Part model, mm, in its own coordinate system. Face numbers are marked on the shaded views. A direction names the side the tool comes from. Give positions to 0.01 mm unless a question says otherwise; leave off trailing zeros. Write each loop counter-clockwise with the first axis right and the second up, starting at its lowest first coordinate (ties: lowest second). Pieces come first, ordered by that corner, then holes.
from build123d import *


with BuildPart() as part:
    # Sketch 1 → Revolve 394 (revolve)
    with BuildSketch(Plane.XY, mode=Mode.PRIVATE) as revolve_394_sk:
        Polygon((-12.5, 0), (-12.5, -37.5), (-10, -37.5), (-10, -207.5), (-12.5, -207.5), (-12.5, -227.5), (0, -227.5), (0, -207.591623727), (-8, -207.591623727), (-8, 0), align=None)
    revolve(revolve_394_sk.sketch.rotate(Axis((0, -1459.557248463, 0), (0, 1, 0)), 180), axis=Axis((0, -1459.557248463, 0), (0, 1, 0)))


with BuildPart() as revolve_813_tool:
    # Sketch 3 → Revolve 813 (revolve)
    with BuildSketch(Plane(origin=(0, 0, 0), x_dir=(1, 0, 0), z_dir=(0, 1, 0))):
        Polygon((-60, 10), (-40, 10), (-36, 10), (-36, 12.5), (36, 12.5), (36, 10), (60, 10), (60, 8), (-60, 8), align=None)
    revolve(axis=Axis((60, 0, 0), (1, 0, 0)))


with BuildPart() as part_1:
    add(part.part)


with BuildPart() as part_2:
    # Revolve 813: joined with revolve_813_tool
    add(part_1.part.fuse(revolve_813_tool.part, tol=0.00001))


solid = part_2.part
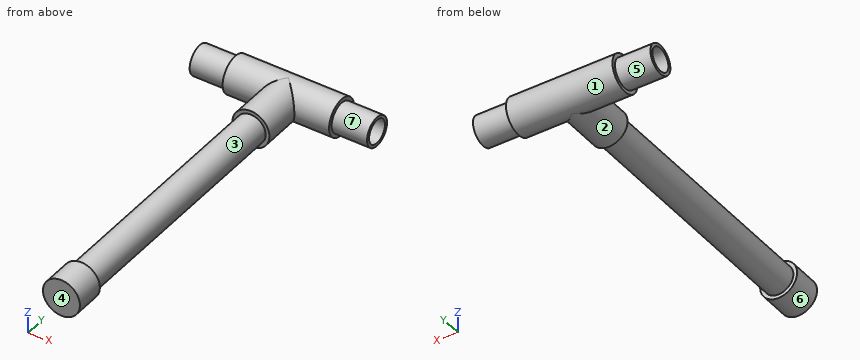
1) Saw through at C-C (z = 0). State how many separate pieces and enclosed holes the cut face has, and give its area (3 significant figures).
Check result:
separate pieces: 2
enclosed holes: 1
area: 2,320 mm2
2) Mould opens along Y. For the marked faces 1, 2, 3 and 4 say: +Y half, -Y half, draft (parallel to the pull), parting line (faces both ways), or undercut.
Check result:
face 1: parting line
face 2: draft
face 3: undercut
face 4: -Y half
3) Flat gauge pins, fed straight in: P1, Ø6, axis at y = -47, z = 0, coming from the +X side; P2, Ø6, axis at y = -26, z = 2, coming from the +X side; P3, Ø8, axis at x = -20.5, z = 5.5, coming from the -Y side. Where does each tip first touch, or does it go through?
Check result:
P1: stops at x = 10
P2: stops at x = 12.5
P3: stops at y = -12.41
4) Drill centre lines: L1, parallel to Z at x = 31, y = 0; L2, parallel to Y at x = 0, z = -1; L3, parallel to Z at x = 0, y = -100. Where is each one in solid material? Low to high.
Check result:
L1: z = -12.5 to -8, 8 to 12.5
L2: y = -227.5 to -207.59, -12.46 to -7.94, 7.94 to 12.46
L3: z = -10 to -8, 8 to 10
5) Saw through at B-B (y = -15). Write the cut outline in (x, z), and give its area (3 significant figures).
Check result:
outline: circle Ø25 at (0, 0); hole circle Ø16 at (0, 0)
area: 290 mm2
6) Saw through at A-A (x = 42). Write the cut outline in (y, z).
Check result:
outline: circle Ø20 at (0, 0); hole circle Ø16 at (0, 0)
7) 3-axis set-ups, long thin cutter, end or side, ignore diameter. For the marked faces 5, 6 and 7: which of +Z, -Z, +X, -X, +Y, -Y reach the whole face in a straight line?
Check result:
face 5: -X
face 6: -Y
face 7: +X
